Study the drawing (mm; zero at the part's minimum x, y, z) and answer. Give positions to 0.01 mm unless a question says otherwise; leave off trailing zeros. Order: outer loops, then holes, each group sorted by start corner. A loop starts at its lowest first (then second) coordinate and runs counter-clockwise, first axis right, second up. Notation, with made-up numbers: (4.5, 83.5) - (9.5, 83.5) arc R28 cw to (9.5, 105.5) - close; hole circle Ø1 at (-36, 61.5). An arc over 180 degrees is marked (long way). Write each question's results on one line, items separated by ' | '. Start each with the question number.
Q1. Flat-ended cylindrical pins translate along their axes: P1, Ø1.5, axis at x = 3, y = 1.5, coming from the -Z side; P2, Ø2.5, axis at x = 15.7, z = 2.5, coming from the +Y side; P3, Ø4, axis at x = 15.7, z = 22.5, coming from the -Y side; P4, Ø0.9, axis at x = 2.5, y = 1.5, coming from the +Z side. Find the tip coordinate at first contact, or state that the pin passes through.
Q2. Find section C-C on z = 17.25. Give the vertices of the cut face in (x, y), and give its area (3 significant figures).
Q3. Find the intervals of material crossed by line 1 along X through (y, z) = (1.4, 13); line 2 along Z through (x, y) = (15.7, 2.45); line 3 along Z through (x, y) = (22.5, 1.9), in increasing order. Write a range as from..to.
Q4. Find section D-D on x = 11.5. Give the vertices of the cut face in (y, z), and give its area (3 significant figures).
Q5. Find section B-B on y = 2.2. Give the vertices of the cut face in (x, z), and give its area (3 significant figures).
Q6. Find section A-A on x = 15.7. Give the vertices of the cut face in (y, z).
Q7. For a pull along X with two mould halves and no side action, classify the marked faces 1, 2, 3 and 4 as +X half, -X half, draft (parallel to the pull), parting line (faces both ways), or undercut.
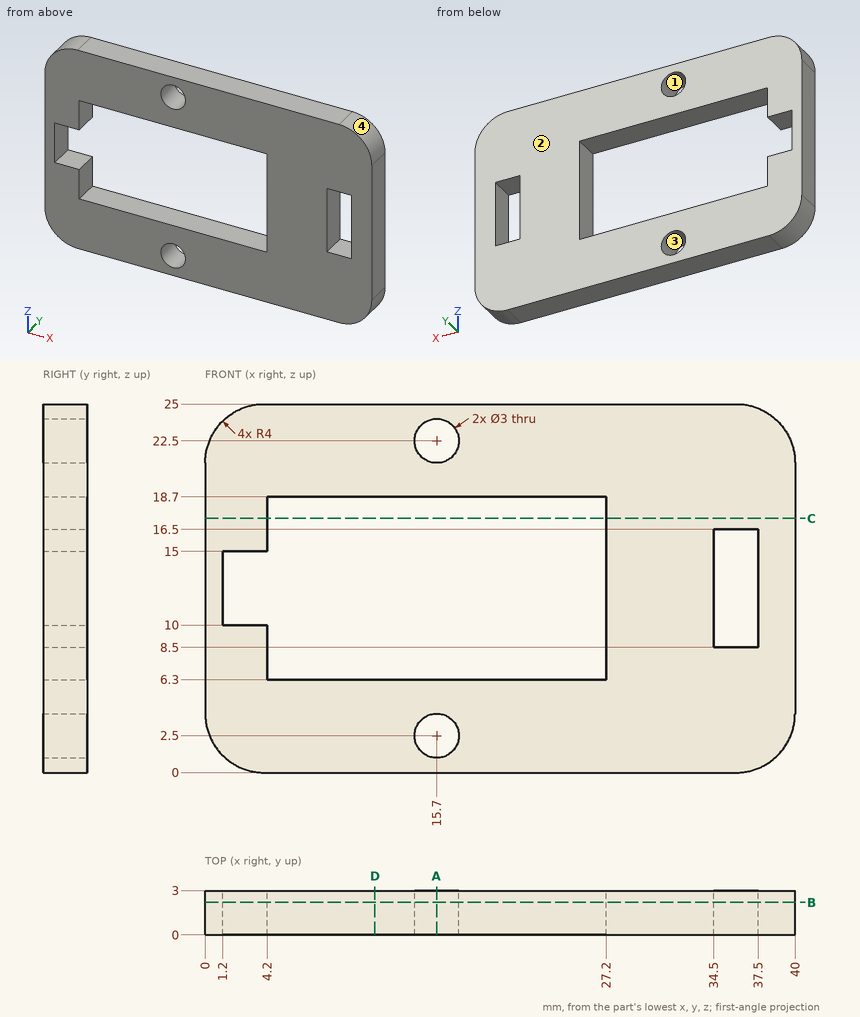
Working result:
1) P1: z = 0.01 | P2: through | P3: y = 0 | P4: z = 24.86
2) outline: (0, 0) - (4.2, 0) - (4.2, 3) - (0, 3) - close; (27.2, 0) - (40, 0) - (40, 3) - (27.2, 3) - close | area: 51.0 mm²
3) line 1: 0..1.2, 27.2..34.5, 37.5..40 | line 2: 0..1, 4..6.3, 18.7..21, 24..25 | line 3: 0..6.3, 18.7..25
4) outline: (0, 0) - (3, 0) - (3, 6.3) - (0, 6.3) - close; (0, 18.7) - (3, 18.7) - (3, 25) - (0, 25) - close | area: 37.8 mm²
5) outline: (0, 4) arc R4 ccw to (4, 0) - (36, 0) arc R4 ccw to (40, 4) - (40, 21) arc R4 ccw to (36, 25) - (4, 25) arc R4 ccw to (0, 21) - close; hole (1.2, 10) - (4.2, 10) - (4.2, 6.3) - (27.2, 6.3) - (27.2, 18.7) - (4.2, 18.7) - (4.2, 15) - (1.2, 15) - close; hole circle Ø3 at (15.7, 2.5); hole circle Ø3 at (15.7, 22.5); hole (34.5, 8.5) - (37.5, 8.5) - (37.5, 16.5) - (34.5, 16.5) - close | area: 648 mm²
6) outline: (0, 0) - (3, 0) - (3, 1) - (0, 1) - close; (0, 4) - (3, 4) - (3, 6.3) - (0, 6.3) - close; (0, 18.7) - (3, 18.7) - (3, 21) - (0, 21) - close; (0, 24) - (3, 24) - (3, 25) - (0, 25) - close
7) face 1: undercut | face 2: draft | face 3: undercut | face 4: +X half
